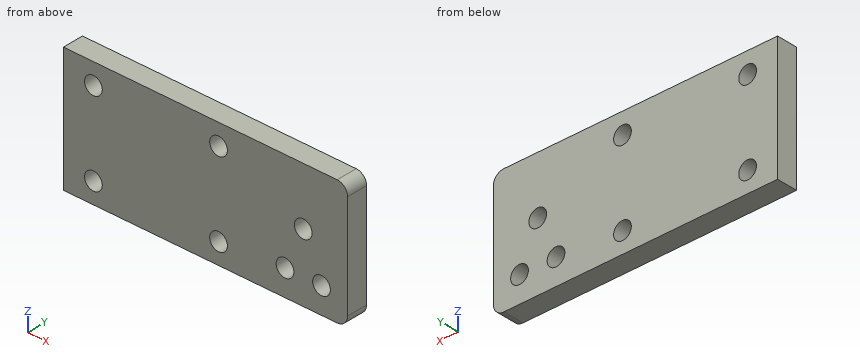
Autodesk Inventor part; units mm, degrees
ref_plane "YZ Plane" through (0, 0, 0) normal (1, 0, 0) x (0, 1, 0)
ref_plane "XZ Plane" through (0, 0, 0) normal (0, 1, 0) x (-1, 0, 0)
ref_plane "XY Plane" through (0, 0, 0) normal (0, 0, 1) x (1, 0, 0)
sketch "Sketch1" plane through (0, 0, 0) normal (0, 1, 0) x (-1, 0, 0)
  line L0 (0, 0) -> (35.5, 0)
  line L1 (35.5, 0) -> (35.5, -24)
  line L2 (35.5, -24) -> (0, -24)
  line L3 (0, -24) -> (0, 0)
  circle A0 centre (5.75, -20) radius 1.7
  circle A1 centre (5.75, -4) radius 1.7
  circle A2 centre (29.75, -20) radius 1.7
  circle A3 centre (29.75, -4) radius 1.7
  line L4 (0, -24) -> (-19, -24)
  line L5 (-19, -24) -> (-19, 0)
  line L6 (-19, 0) -> (0, 0)
  line L7 (0, 0) -> (0, -24)
  circle A4 centre (-14, -19) radius 1.7
  circle A5 centre (-7, -19) radius 1.7
  circle A6 centre (-10.5, -11) radius 1.7
  line L8 (35.5, -24) -> (35.5, 0)
  dimension "d0" = 35.5
  dimension "d1" = 24
  dimension "d2" = 3.4
  dimension "d3" = 4
  dimension "d4" = 5.75
  dimension "d5" = 3.4
  dimension "d6" = 16
  dimension "d7" = 3.4
  dimension "d8" = 4
  dimension "d9" = 5.75
  dimension "d10" = 3.4
  dimension "d11" = 16
  dimension "d12" = 19
  dimension "d13" = 24
  dimension "d14" = 3.4
  dimension "d15" = 5
  dimension "d16" = 5
  dimension "d17" = 3.4
  dimension "d18" = 7
  dimension "d19" = 3.4
  dimension "d20" = 8
  dimension "d21" = 3.5
  dimension "d35" = 24
extrude "Extrusion1" add sketch "Sketch1" along normal blind 4
fillet "Fillet1" radius 2 2 edges at (19, 2, 0) (19, 2, -24)
properties part number "drag chain mount"
Can you work these out from the model? Positions are in its coordinate system, mm. Give positions to 0.01 mm unless a question says otherwise; leave off trailing zeros. Loops run counter-clockwise (first coordinate to the right, second up) from the corner with the lowest first, then second, coordinate; pieces in that order, holes last. Notation, with made-up numbers: M 57,80.25 L 113,80.25 A13 cw 113,94.25 Z; hole C -32.5,13 d9. An arc over 180 degrees is marked long. One line per item, written item: value.
(1) Suppose I cut it at B-B on x = 10.5. List the corners of the cut face in (y, z) for me, plus the area to 3 significant figures.
Returned:
outline: M 0,-24 L 4,-24 L 4,-12.7 L 0,-12.7 Z; M 0,-9.3 L 4,-9.3 L 4,0 L 0,0 Z
area: 82.4 mm^2
(2) Suppose I cut it at A-A on x = -5.75. List the corners of the cut face in (y, z) for me, plus the area to 3 significant figures.
Returned:
outline: M 0,-24 L 4,-24 L 4,-21.7 L 0,-21.7 Z; M 0,-18.3 L 4,-18.3 L 4,-5.7 L 0,-5.7 Z; M 0,-2.3 L 4,-2.3 L 4,0 L 0,0 Z
area: 68.8 mm^2
(3) Will this pin go through, and if not, where does the flat tip stop? pin 1 (3 mm diameter, centred on x = 10.5, z = -11, fed in from -Y).
Returned:
pin 1: through
(4) Suppose I cut it at C-C on z = -10.5. List the corners of the cut face in (x, y) for me, plus the area to 3 significant figures.
Returned:
outline: M -35.5,0 L 8.88,0 L 8.88,4 L -35.5,4 Z; M 12.12,0 L 19,0 L 19,4 L 12.12,4 Z
area: 205 mm^2
(5) Suppose I cut it at D-D on y = 0.55. List the corners of the cut face in (x, z) for me.
Returned:
outline: M -35.5,-24 L 17,-24 A2 ccw 19,-22 L 19,-2 A2 ccw 17,0 L -35.5,0 Z; hole C -29.75,-20 d3.4; hole C -29.75,-4 d3.4; hole C -5.75,-20 d3.4; hole C -5.75,-4 d3.4; hole C 7,-19 d3.4; hole C 10.5,-11 d3.4; hole C 14,-19 d3.4
(6) I need wall thicknesses on line 1 (Z direction, x = -29.75, y = 1.3); line 2 (Z direction, x = 14, y = 2.45); line 3 (Z direction, x = 10.5, y = 2.5). Which ranges of each line are inside material? Lowest first, please.
Returned:
line 1: -24 to -21.7, -18.3 to -5.7, -2.3 to 0
line 2: -24 to -20.7, -17.3 to 0
line 3: -24 to -12.7, -9.3 to 0
